Source: CAD feature listing. Evaluate the final solid. Frame: model axes, mm. Face numbers are marked on the shaded views. A direction names the side the tool comes from. Round coordinates to 2 decimals unless told otherwise and drop trailing zeros. Write each loop counter-clockwise with the first axis right and the second up, starting at its lowest first coordinate (ties: lowest second). Pieces come first, ordered by that corner, then holes. Notation, with made-up numbers: M 54.5,72.5 L 84.5,72.5 A22 cw 84.5,80.5 Z; hole C 65,-39 d4. An arc over 180 degrees is marked long. Put each result on its own line as item: value. Start each with the question number.
```python
from build123d import *

# Parameters (mm, degrees)
SKETCH1_W               = 50
SKETCH1_H               = 44
BASE_FLANGE1_DEPTH      = 2
EDGE_FLANGE1_DEPTH      = 44
EDGE_FLANGE1_BEND_DEPTH = 44
EDGE_FLANGE2_DEPTH      = 44
EDGE_FLANGE2_BEND_DEPTH = 44
SKETCH21_R              = 12.5
SKETCH21_R_2            = 2.25
CUT_EXTRUDE1_DEPTH      = 2
SKETCH22_R              = 2
CUT_EXTRUDE2_DEPTH      = 2
FILLET1_R               = 4


# Sheet-metal steps are written as plain solids
with BuildPart() as part:
    # Sketch1 → Base-Flange1 (new body)
    with BuildSketch(Plane(origin=(0, 0, 0), x_dir=(1, 0, 0), z_dir=(0, 1, 0))):
        with Locations((45, -1)):
            Rectangle(SKETCH1_W, SKETCH1_H)
    extrude(amount=-BASE_FLANGE1_DEPTH)

    # Edge-Flange1 section (across the edge) → Edge-Flange1 (add)
    with BuildSketch(Plane(origin=(18.8, 0, -21), x_dir=(1, 0, 0), z_dir=(0, 0, 1))):
        with BuildLine():
            Line((-2, 1.2), (-2, 38))
            Line((-2, 38), (0, 38))
            Line((0, 38), (0, 1.2))
            ThreePointArc((0, 1.2), (0.351471863, 0.351471863), (1.2, 0))
            Line((1.2, 0), (1.2, -2))
            ThreePointArc((1.2, -2), (-1.0627417, -1.0627417), (-2, 1.2))
        make_face()
    extrude(amount=EDGE_FLANGE1_DEPTH)

    # Edge-Flange1 section 2 (across the edge) → Edge-Flange1 bend (add)
    with BuildSketch(Plane(origin=(71.2, 0, 23), x_dir=(-1, 0, 0), z_dir=(0, 0, -1))):
        with BuildLine():
            Line((-2, 1.2), (-2, 38))
            Line((-2, 38), (0, 38))
            Line((0, 38), (0, 1.2))
            ThreePointArc((0, 1.2), (0.351471863, 0.351471863), (1.2, 0))
            Line((1.2, 0), (1.2, -2))
            ThreePointArc((1.2, -2), (-1.0627417, -1.0627417), (-2, 1.2))
        make_face()
    extrude(amount=EDGE_FLANGE1_BEND_DEPTH)

    # Edge-Flange2 section (across the edge) → Edge-Flange2 (add)
    with BuildSketch(Plane(origin=(73.2, 39.2, -21), x_dir=(0, -1, 0), z_dir=(0, 0, 1))):
        with BuildLine():
            Line((-2, 1.2), (-2, 16))
            Line((-2, 16), (0, 16))
            Line((0, 16), (0, 1.2))
            ThreePointArc((0, 1.2), (0.351471863, 0.351471863), (1.2, 0))
            Line((1.2, 0), (1.2, -2))
            ThreePointArc((1.2, -2), (-1.0627417, -1.0627417), (-2, 1.2))
        make_face()
    extrude(amount=EDGE_FLANGE2_DEPTH)

    # Edge-Flange2 section 2 (across the edge) → Edge-Flange2 bend (add)
    with BuildSketch(Plane(origin=(16.8, 39.2, 23), x_dir=(0, -1, 0), z_dir=(0, 0, -1))):
        with BuildLine():
            Line((-2, 1.2), (-2, 16))
            Line((-2, 16), (0, 16))
            Line((0, 16), (0, 1.2))
            ThreePointArc((0, 1.2), (0.351471863, 0.351471863), (1.2, 0))
            Line((1.2, 0), (1.2, -2))
            ThreePointArc((1.2, -2), (-1.0627417, -1.0627417), (-2, 1.2))
        make_face()
    extrude(amount=EDGE_FLANGE2_BEND_DEPTH)

    # Sketch21 → Cut-Extrude1 (cut)
    with BuildSketch(Plane.XZ.offset(2)):
        with Locations(Location((45, 1, 0), (0, 0, 270))):
            Circle(SKETCH21_R)
        with Locations(Location((57.02081528, 13.02081528, 0), (0, 0, 270))):
            Circle(SKETCH21_R_2)
        with Locations(Location((57.02081528, -11.02081528, 0), (0, 0, 270))):
            Circle(SKETCH21_R_2)
        with Locations(Location((32.97918472, -11.02081528, 0), (0, 0, 270))):
            Circle(SKETCH21_R_2)
        with Locations(Location((32.97918472, 13.02081528, 0), (0, 0, 270))):
            Circle(SKETCH21_R_2)
    extrude(amount=-CUT_EXTRUDE1_DEPTH, mode=Mode.SUBTRACT)

    # Sketch22 → Cut-Extrude2 (cut)
    with BuildSketch(Plane.XZ.offset(-39.2)):
        with Locations(Location((8.2, 18, 0), (0, 0, 270))):
            Circle(SKETCH22_R)
        with Locations(Location((8.2, -16, 0), (0, 0, 270))):
            Circle(SKETCH22_R)
        with Locations(Location((81.8, -16, 0), (0, 0, 90))):
            Circle(SKETCH22_R)
        with Locations(Location((81.8, 18, 0), (0, 0, 90))):
            Circle(SKETCH22_R)
    extrude(amount=-CUT_EXTRUDE2_DEPTH, mode=Mode.SUBTRACT)

    # Fillet1
    fillet1_edges = [part.edges().sort_by_distance(p)[0] for p in [
        (89.2, 40.2, -21),
        (89.2, 40.2, 23),
        (0.8, 40.2, 23),
        (0.8, 40.2, -21),
    ]]
    fillet(fillet1_edges, radius=FILLET1_R)


solid = part.part
```
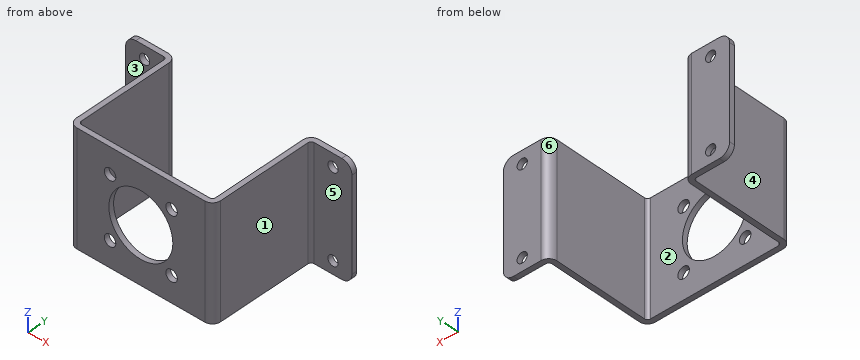
(1) Section query A-A (z = 18). Return loops of the section in (x, y), and give its area (3 significant figures).
(2) Ray query, line 1 along Z through (x, y) = (81, 40); line 2 along X through (y, z) = (40, 18); line 3 along X through (y, z) = (12.5, -8.5). Return the intervals inside material, ascending.
(3) Access query for the marked faces 4, 5 and 6. Directions: +Z, -Z, +X, -X, +Y, -Y. A direction counts if a zero-diameter tool reaches every point of the face in a straight line with its end or side. Return the directions, or none.
(4) Section query C-C (x = 8.2). Return loops of the section in (y, z).
(5) Pull-direction query (X, two-part tool) for the marked faces 1, 2 and 3; classes: +X half, -X half, draft (parallel to the pull), parting line (faces both ways), or undercut.
(6) Section query B-B (y = 5). Return loops of the section in (x, z), and give its area (3 significant figures).
(7) Section query D-D (x = 45). Return loops of the section in (y, z).
(8) Contact query for flat-ended pins moving along their axis: P1, Ø4.5, axis at x = 5.5, z = 11.5, coming from the -Y side; P2, Ø11, axis at y = 24.5, z = 9.5, coming from the -X side; P3, Ø2, axis at y = 16.5, z = -11, coming from the +X side. Output: stop coordinate, or through.
Entries:
1. outline: M 0.8,39.2 L 6.2,39.2 L 6.2,41.2 L 0.8,41.2 Z; M 10.2,39.2 L 15.6,39.2 A1.2 cw 16.8,38 L 16.8,1.2 A3.2 ccw 20,-2 L 70,-2 A3.2 ccw 73.2,1.2 L 73.2,38 A1.2 cw 74.4,39.2 L 79.8,39.2 L 79.8,41.2 L 74.4,41.2 A3.2 ccw 71.2,38 L 71.2,1.2 A1.2 cw 70,0 L 20,0 A1.2 cw 18.8,1.2 L 18.8,38 A3.2 ccw 15.6,41.2 L 10.2,41.2 Z; M 83.8,39.2 L 89.2,39.2 L 89.2,41.2 L 83.8,41.2 Z
1. area: 318 mm2
2. line 1: -21 to -17.83, -14.17 to 16.17, 19.83 to 23
2. line 2: 0.8 to 6.2, 10.2 to 18.1, 71.9 to 79.8, 83.8 to 89.2
2. line 3: 16.8 to 18.8, 71.2 to 73.2
3. face 4: +Z, -Z, -X, -Y
3. face 5: +Z, -Z, +X, -Y
3. face 6: +Z, -Z, +Y
4. outline: M 39.2,-21 L 41.2,-21 L 41.2,-18 L 39.2,-18 Z; M 39.2,-14 L 41.2,-14 L 41.2,16 L 39.2,16 Z; M 39.2,20 L 41.2,20 L 41.2,23 L 39.2,23 Z
5. face 1: +X half
5. face 2: undercut
5. face 3: draft
6. outline: M 16.8,-21 L 18.8,-21 L 18.8,23 L 16.8,23 Z; M 71.2,-21 L 73.2,-21 L 73.2,23 L 71.2,23 Z
6. area: 176 mm2
7. outline: M -2,-21 L 0,-21 L 0,-11.5 L -2,-11.5 Z; M -2,13.5 L 0,13.5 L 0,23 L -2,23 Z
8. P1: y = 39.2
8. P2: x = 16.8
8. P3: x = 73.2
